Can you work these out from the model? Positions are in its coordinate system, mm. Face numbers are marked on the shaded views. A direction names the side the tool comes from. Round coordinates to 2 decimals unless told otherwise and drop trailing zeros. Loops run counter-clockwise (first coordinate to the right, second up) from the corner with the lowest first, then second, coordinate; pieces in that order, holes last.
(1) Which directions (+Z, -Z, +X, -X, +Y, -Y) give clear straight access to the entire face, cutting with the end or side of a thin tool? Please do the marked faces 1 and 2.
(2) I want a section at A-A on x = 37. Write out the boundary of the cut face in (y, z).
(3) I want a section at C-C on y = 46.5. Write out the boundary of the cut face in (x, z).
(4) I want a section at B-B on z = 1.7. Write out the boundary of the cut face in (x, y), plus the area to 3 significant figures.
(5) Will these pins go through, and if not, where does the flat tip stop? pin 1 Ø1.5 at (y, z) = (42.5, 2) entering from -X; pin 2 Ø1.8 at (x, y) = (42.4, 42.38) entering from -Z.
(6) I want a section at D-D on x = 47. Write out the boundary of the cut face in (y, z).
(7) If I drill on line 1 along Y through (x, z) = (42.4, 0.65); line 2 along X through (y, z) = (42, 2.35); line 3 along X through (y, z) = (43.75, 0.85), over which ranges is the centre line in solid material (lowest first)?
(8) Thinking about a two-plate mould opening in Y: for the marked faces 3, 4 and 5, which applies, released by +Y, released by -Y, zero draft, split by the parting line, or undercut?
from build123d import *

# Parameters (mm, degrees)
CORTE_EXTERIOR_R        = 1
SALIENTE_EXTRUIR1_DEPTH = 3


with BuildPart() as part:
    # Corte exterior → Saliente-Extruir1 (new body)
    with BuildSketch(Plane.XY):
        with BuildLine():
            Line((42.4, 49.878566683), (34.6, 49.878566683))
            Line((34.6, 49.878566683), (34.6, 44.878566683))
            Line((34.6, 44.878566683), (37.6, 44.878566683))
            Line((37.6, 44.878566683), (37.6, 39.878566683))
            Line((37.6, 39.878566683), (34.6, 39.878566683))
            Line((34.6, 39.878566683), (34.6, 34.878566683))
            Line((34.6, 34.878566683), (42.4, 34.878566683))
            ThreePointArc((42.4, 34.878566683), (49.9, 42.378566683), (42.4, 49.878566683))
        make_face()
        with Locations((42.4, 42.378566683)):
            Circle(CORTE_EXTERIOR_R, mode=Mode.SUBTRACT)
    extrude(amount=SALIENTE_EXTRUIR1_DEPTH)


solid = part.part
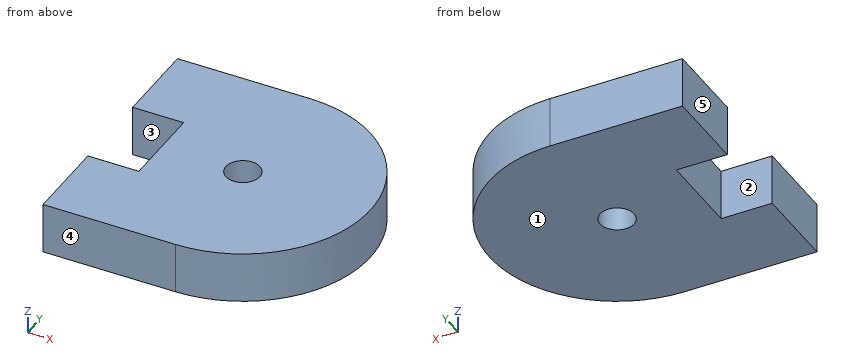
Filled sheet:
1. face 1: -Z, +X, -X, +Y, -Y
1. face 2: +Z, -Z, -X
2. outline: (34.88, 0) - (39.88, 0) - (39.88, 3) - (34.88, 3) - close; (44.88, 0) - (49.88, 0) - (49.88, 3) - (44.88, 3) - close
3. outline: (34.6, 0) - (48.67, 0) - (48.67, 3) - (34.6, 3) - close
4. outline: (34.6, 34.88) - (42.4, 34.88) arc R7.5 ccw to (42.4, 49.88) - (34.6, 49.88) - (34.6, 44.88) - (37.6, 44.88) - (37.6, 39.88) - (34.6, 39.88) - close; hole circle Ø2 at (42.4, 42.38)
4. area: 187 mm2
5. pin 1: stops at x = 37.6
5. pin 2: passes through
6. outline: (36.45, 0) - (48.3, 0) - (48.3, 3) - (36.45, 3) - close
7. line 1: y = 34.88 to 41.38, 43.38 to 49.88
7. line 2: x = 37.6 to 41.47, 43.33 to 49.89
7. line 3: x = 37.6 to 49.77
8. face 3: undercut
8. face 4: released by -Y
8. face 5: zero draft
